```python
from build123d import *

# Parameters (mm, degrees)
F2_W            = 26.7493221909
F2_H            = 40.8729631454
F3_DEPTH        = 25
F3_DEPTH_BACK   = 37.9
F6_R            = 0.75
F7_DEPTH        = 2.5
F7_COPIES_COUNT = 3


# Not quite as in the source:
# - a pattern or mirror of a feature is missing from the dataset's text; its kind, count and spacing are read off the source's solid


with BuildPart() as f1:
    # F0 (on Top) → F1 (revolve)
    with BuildSketch(Plane.XY):
        with BuildLine():
            Line((0, 11.5), (0, -11.5))
            ThreePointArc((0, -11.5), (11.5, 0), (0, 11.5))
        make_face()
    revolve(axis=Axis((0, 0, 0), (0, -1, 0)))

    # F2 (on Top) → F3 (cut, two sides)
    with BuildSketch(Plane.XY) as f3_sk:
        with Locations((13.3746610954, -0.1069968566)):
            Rectangle(F2_W, F2_H)
    extrude(amount=-F3_DEPTH, mode=Mode.SUBTRACT)
    extrude(f3_sk.sketch, amount=F3_DEPTH_BACK, mode=Mode.SUBTRACT)

    # F4 (on face) → F5 (revolve, cut)
    with BuildSketch(Plane.YZ):
        with BuildLine():
            Line((0, 9.5), (0, -9.5))
            ThreePointArc((0, -9.5), (9.5, 0), (0, 9.5))
        make_face()
    revolve(axis=Axis((0, 0, 0), (0, 0, -1)), mode=Mode.SUBTRACT)

    # F6 (on face) → F7 (join)
    with BuildSketch(Plane.YZ):
        with Locations((-9.2580689408, 4.9536006588)):
            Circle(F6_R)
    f7 = extrude(amount=F7_DEPTH)

    # F7_copies: F7 ×3 about axis
    f7_copies_axis = Axis((0, 0, 0), (1, 0, 0))
    for i in range(1, F7_COPIES_COUNT):
        add(f7.rotate(f7_copies_axis, i * 360 / F7_COPIES_COUNT))


solid = f1.part
```
Could you check a few things on this model? Use its own coordinates, in mm. Round coordinates to 2 decimals unless told otherwise and drop trailing zeros. Loops run counter-clockwise (first coordinate to the right, second up) from the corner with the lowest first, then second, coordinate; pieces in that order, holes last.
Q1. Please list where these lines run through material, in increasing order: L1, parallel to Z at x = -1.5, y = 1.75; L2, parallel to Z at x = -4.5, y = -0.5; L3, parallel to Y at x = -2.75, z = 7.75.
Q2. I want a section at A-A (x = 0.75). Write out the boundary of the cut face in (y, z) (3 decimals), and give its area (3 significant figures).
Q3. I want a section at D-D (y = -8). Write out the boundary of the cut face in (x, z).
Q4. I want a section at B-B (x = -3). Write out the boundary of the cut face in (y, z).
Q5. I want a section at C-C (z = 3). Write out the boundary of the cut face in (x, y).
Q6. For P1, Ø3, axis at x = -3.5, y = -4, coming from the -Z side; P2, Ø6, axis at y = 4.5, z = 0, coming from the +X side; P3, Ø4, axis at x = 0.5, z = -9, coming from the +Y side, each with a flat end and sliding along its axis, tell me the tip position at first contact or that it passes through.
Q7. Thinking about a two-plate mould opening in Y: for faces 1 (the flat face through (2.5, 9, 6)), 2 (the cylindrical face through (1.232, -8.543, 5.179)), 3 (the cylindrical face through (1.23, 9.61, 5.25)), 4 (the cylindrical face through (1.232, 0.177, -11.227)), which applies, pulls with the +Y half, pulls with the -Y half, needs draft (parallel to the pull), parting line crosses it, or undercut?
Answer below:
1. L1: z = -11.27 to -9.22, 9.22 to 11.27
1. L2: z = -10.57 to -8.35, 8.35 to 10.57
1. L3: y = -8.04 to -4.76, 4.76 to 8.04
2. outline: circle Ø1.5 at (-9.258, 4.954); circle Ø1.5 at (0.339, -10.495); circle Ø1.5 at (8.919, 5.541)
2. area: 5.30 mm2
3. outline: (0, -8.26) - (0, -5.12) arc R5.12 cw to (0, 5.12) - (0, 8.26) arc R8.26 ccw to start
4. outline: circle Ø22.2 at (0, 0); hole circle Ø18.03 at (0, 0)
5. outline: (0, -11.1) - (0, -9.01) arc R9.01 cw to (0, 9.01) - (0, 11.1) arc R11.1 ccw to start
6. P1: stops at z = -10.85
6. P2: stops at x = -5.83
6. P3: stops at y = 9.08
7. face 1: needs draft
7. face 2: undercut
7. face 3: undercut
7. face 4: parting line crosses it
